Geometry check sheet. Reference: the model listing, model coordinates, mm. Face numbers are marked on the shaded views. A direction names the side the tool comes from. Give positions to 0.01 mm unless a question says otherwise; leave off trailing zeros. Loops run counter-clockwise (first coordinate to the right, second up) from the corner with the lowest first, then second, coordinate; pieces in that order, holes last. Notation, with made-up numbers: (-39.75, 39) -> (-20.75, 39) arc R16 cw to (-20.75, 53) -> close; hole circle Ø3 at (9.25, 32.25). An arc over 180 degrees is marked (long way). One line per question, with ' | ' between items.
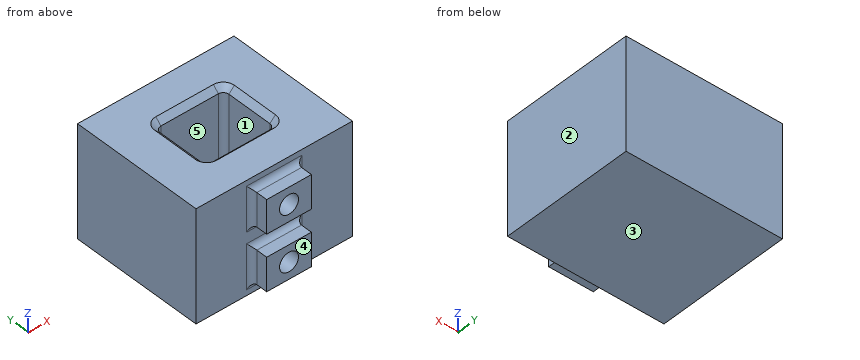
from build123d import *

# Parameters (mm, degrees)
SKETCH1_W           = 28
SKETCH1_H           = 24
BOSS_EXTRUDE1_DEPTH = 20
SKETCH2_W           = 12.3
SKETCH2_H           = 10.3
CUT_EXTRUDE1_DEPTH  = 15.3
SKETCH3_W           = 8
SKETCH3_H           = 6
SKETCH3_R           = 1.7
BOSS_EXTRUDE3_DEPTH = 3
FILLET1_R           = 1
CHAMFER1_SIZE       = 1
FILLET2_R           = 1


with BuildPart() as part:
    # Sketch1 → Boss-Extrude1 (new body)
    with BuildSketch(Plane.XY):
        Rectangle(SKETCH1_W, SKETCH1_H)
    extrude(amount=BOSS_EXTRUDE1_DEPTH)

    # Sketch2 → Cut-Extrude1 (cut)
    with BuildSketch(Plane.XY.offset(20)):
        Rectangle(SKETCH2_W, SKETCH2_H)
    extrude(amount=-CUT_EXTRUDE1_DEPTH, mode=Mode.SUBTRACT)

    # Sketch3 → Boss-Extrude3 (add)
    # profile 1 of 2: a face of its own
    with BuildSketch(Plane.XZ.offset(12)):
        with Locations((0, 5)):
            Rectangle(SKETCH3_W, SKETCH3_H)
        with Locations(Location((0, 5, 0), (0, 0, 90))):
            Circle(SKETCH3_R, mode=Mode.SUBTRACT)
    # profile 2 of 2: a face of its own
    with BuildSketch(Plane.XZ.offset(12)):
        with Locations((0, 15)):
            Rectangle(SKETCH3_W, SKETCH3_H)
        with Locations(Location((0, 15, 0), (0, 0, 270))):
            Circle(SKETCH3_R, mode=Mode.SUBTRACT)
    extrude(amount=BOSS_EXTRUDE3_DEPTH)

    # Fillet1
    fillet1_edges = [part.edges().sort_by_distance(p)[0] for p in [
        (-6.15, 5.15, 12.35),
        (6.15, 5.15, 12.35),
        (6.15, -5.15, 12.35),
        (-6.15, -5.15, 12.35),
    ]]
    fillet(fillet1_edges, radius=FILLET1_R)

    # Chamfer1
    chamfer1_edges = [part.edges().sort_by_distance(p)[0] for p in [
        (6.15, 0, 20),
        (0, -5.15, 20),
        (0, 5.15, 20),
        (-6.15, 0, 20),
        (5.857106781, -4.857106781, 20),
        (5.857106781, 4.857106781, 20),
        (-5.857106781, 4.857106781, 20),
        (-5.857106781, -4.857106781, 20),
    ]]
    chamfer(chamfer1_edges, length=CHAMFER1_SIZE)

    # Fillet2
    fillet2_edges = [part.edges().sort_by_distance(p)[0] for p in [
        (4, -12, 15),
        (0, -12, 18),
        (-4, -12, 15),
        (0, -12, 12),
        (-4, -12, 5),
        (0, -12, 2),
        (4, -12, 5),
        (0, -12, 8),
    ]]
    fillet(fillet2_edges, radius=FILLET2_R)


solid = part.part
Item 1: Scan lines: probe 1 along X at (y, z) = (3.5, 12); probe 2 along Y at (x, z) = (1.75, 5.75). Record each from-to range of solid material in increasing order.
Result:
probe 1: -14 to -6.15, 6.15 to 14 | probe 2: -15 to -5.15, 5.15 to 12
Item 2: Set-up check for the marked faces 4 and 5: record each of +Z, -Z, +X, -X, +Y, -Y from which the full face is reachable in a straight line by a thin tool's end or side.
Result:
face 4: +Z, -Z, +X, -X, -Y | face 5: +Z
Item 3: Sectioned sample at B-B (y = -1.5). Record the cut outline in (x, z), plus the area to 3 significant figures.
Result:
outline: (-14, 0) -> (14, 0) -> (14, 20) -> (7.15, 20) -> (6.15, 19) -> (6.15, 4.7) -> (-6.15, 4.7) -> (-6.15, 19) -> (-7.15, 20) -> (-14, 20) -> close | area: 371 mm2
Item 4: Sectioned sample at A-A (z = 10.25). Record the cut outline in (x, y), plus the area to 3 significant figures.
Result:
outline: (-14, -12) -> (14, -12) -> (14, 12) -> (-14, 12) -> close; hole (-6.15, -4.15) arc R1 ccw to (-5.15, -5.15) -> (5.15, -5.15) arc R1 ccw to (6.15, -4.15) -> (6.15, 4.15) arc R1 ccw to (5.15, 5.15) -> (-5.15, 5.15) arc R1 ccw to (-6.15, 4.15) -> close | area: 546 mm2
Item 5: Release check for a two-part mould opening along X. For the marked faces 1, 2 and 3 record: pulls with the +X half, pulls with the -X half, needs draft (parallel to the pull), parting line crosses it, or undercut.
Result:
face 1: undercut | face 2: pulls with the +X half | face 3: needs draft
Item 6: Sectioned sample at D-D (z = 15). Record the cut outline in (x, y), plus the area to 3 significant figures.
Result:
outline: (-14, -12) -> (-5, -12) arc R1 cw to (-4, -13) -> (-4, -15) -> (-1.7, -15) -> (-1.7, -12) -> (1.7, -12) -> (1.7, -15) -> (4, -15) -> (4, -13) arc R1 cw to (5, -12) -> (14, -12) -> (14, 12) -> (-14, 12) -> close; hole (-6.15, -4.15) arc R1 ccw to (-5.15, -5.15) -> (5.15, -5.15) arc R1 ccw to (6.15, -4.15) -> (6.15, 4.15) arc R1 ccw to (5.15, 5.15) -> (-5.15, 5.15) arc R1 ccw to (-6.15, 4.15) -> close | area: 560 mm2
Item 7: Depth check by flat-ended pin: pin 1 Ø5 at (x, y) = (1, -2.5) entering from +Z; pin 2 Ø1.7 at (x, z) = (0.5, 5) entering from -Y; pin 3 Ø12 at (x, z) = (1.5, 10.5) entering from -Y; pin 4 Ø1 at (x, y) = (-1.5, -14.5) entering from +Z. Enter the tip coordinate at first touch or a pass-through.
Result:
pin 1: z = 4.7 | pin 2: y = -12 | pin 3: y = -15 | pin 4: z = 18
